Input: part model. Units: mm. Frame: model coordinates. A direction names the side the tool comes from. Give positions to 0.01 mm unless a question says otherwise; leave off trailing zeros. Loops run counter-clockwise (first coordinate to the right, second up) from the corner with the lowest first, then second, coordinate; pieces in that order, holes last. Notation, with made-up numbers: M 25,-13.75 L 56,-13.75 A10 ccw 56,-7.75 Z; hole C 21.25,53.5 d5. An arc over 180 degrees is marked long. One line per item, written item: value. Start each with the question number.
(1) Section C-C on y = -43. Output: boundary loops of the cut face in (x, z), plus the area to 3 significant figures.
(2) Ray query, line 1 along Z through (x, y) = (-49, -48.5); line 2 along X through (y, z) = (-38, -69.5); line 3 along Y through (x, z) = (35.5, 12.5). Return the intervals inside material, ascending. Write a range as from..to.
(3) Section D-D on y = -85.5. Output: boundary loops of the cut face in (x, z).
(4) Section B-B on x = 57.5. Output: boundary loops of the cut face in (y, z), plus the area to 3 significant figures.
(5) Section A-A on z = -60.5. Output: boundary loops of the cut face in (x, y), plus the area to 3 significant figures.
(6) Pin query (flat end, axial travel): P1, Ø3.5, axis at x = -70, z = -70.5, coming from the -Y side; P2, Ø5, axis at x = 2.66, y = -73.34, coming from the +Z side. Return the tip coordinate at first contact, or that it passes through.
(7) Pull-direction query (Y, two-part tool) for faces 1 (the flat face through (-69, -52.086, -56)), 2 (the flat face through (1, -70, -130)), 3 (the cylindrical face through (-3.626, -178.175, -120.14)), 4 (the cylindrical face through (48.677, -115.843, 9.86)); classes: released by +Y, released by -Y, zero draft, split by the parting line, or undercut.
(8) Access query for faces 5 (the flat face through (-1, -22.086, 13)), 6 (the flat face through (70, -195, 10)), 7 (the flat face through (1, -70, -110)), 8 (the flat face through (-63, -37, -54)), 9 (the flat face through (69, -52.086, -56)). Directions: +Z, -Z, +X, -X, +Y, -Y. A direction counts if a zero-diameter tool reaches every point of the face in a straight line with its end or side. Return the directions, or none.
```python
from build123d import *

# Parameters (mm, degrees)
EXTRUDE_1_OUTLINE_W     = 150
EXTRUDE_1_OUTLINE_H     = 400
EXTRUDE_1_OUTLINE_R     = 48.25
EXTRUDE_1_DEPTH         = 20
SKETCH_2_W              = 150
SKETCH_2_H              = 400
SKETCH_2_W_2            = 126
SKETCH_2_H_2            = 376
EXTRUDE_1_2_DEPTH       = 110
EXTRUDE_START           = 20
SKETCH_3_W              = 150
SKETCH_3_H              = 400
SKETCH_3_R              = 48.25
EXTRUDE_3_DEPTH         = 20
SKETCH_4_W              = 110
SKETCH_4_H              = 55
CUT_EXTRUDE_1_DEPTH     = 428.229446551
CHAMFER_2_SIZE          = 20
CHAMFER_3_SIZE          = 20
CUT_EXTRUDE_START       = 190
CUT_EXTRUDE_2_OUTLINE_W = 132
CUT_EXTRUDE_2_OUTLINE_H = 152
CUT_EXTRUDE_2_DEPTH     = 10
FILLET_1_R              = 20
FILLET_2_R              = 20
FILLET_3_R              = 20
FILLET_4_R              = 20
EXTRUDE_START_2         = -20
SKETCH_6_R              = 48.25
SKETCH_6_R_2            = 29.5
EXTRUDE_4_DEPTH         = 20
SKETCH_7_R              = 48.25
SKETCH_7_R_2            = 29.5
EXTRUDE_5_DEPTH         = 20
SKETCH_8_R              = 29.5
EXTRUDE_7_DEPTH         = 20
SKETCH_9_R              = 29.5
EXTRUDE_8_DEPTH         = 20
SKETCH_10_R             = 1.65
EXTRUDE_9_DEPTH         = 10
EXTRUDE_START_3         = 10
SKETCH_11_R             = 1.65
EXTRUDE_10_DEPTH        = 10
SKETCH_12_W             = 110
SKETCH_12_H             = 147.914448675
CUT_EXTRUDE_3_DEPTH     = 287.530975638
CHAMFER_4_SIZE          = 10
CHAMFER_5_SIZE          = 10
SKETCH_13_W             = 150
SKETCH_13_H             = 80
CUT_EXTRUDE_5_DEPTH     = 267.880122902
CUT_EXTRUDE_6_REACH     = 263.008
SKETCH_15_R             = 1.5
SKETCH_16_R             = 1.5
CUT_EXTRUDE_7_DEPTH     = 262.007662723


with BuildPart() as part:
    # Extrude 1: read off the stored shape, not the designer's step
    # Extrude 1 outline → Extrude 1 (new body)
    with BuildSketch(Plane.XY):
        Rectangle(EXTRUDE_1_OUTLINE_W, EXTRUDE_1_OUTLINE_H)
        with Locations((2.655190842, -130.335551325)):
            Circle(EXTRUDE_1_OUTLINE_R, mode=Mode.SUBTRACT)
        with Locations((0, 129.13990983)):
            Circle(EXTRUDE_1_OUTLINE_R, mode=Mode.SUBTRACT)
    extrude(amount=EXTRUDE_1_DEPTH)

    # 草图2 → Extrude 1 2 (add)
    with BuildSketch(Plane(origin=(0, 0, 0), x_dir=(-1, 0, 0), z_dir=(0, 0, -1))):
        Rectangle(SKETCH_2_W, SKETCH_2_H)
        Rectangle(SKETCH_2_W_2, SKETCH_2_H_2, mode=Mode.SUBTRACT)
    extrude(amount=EXTRUDE_1_2_DEPTH)

    # 草图3 → 凸台-拉伸3 (add)
    with BuildSketch(Plane(origin=(0, 0, -110), x_dir=(-1, 0, 0), z_dir=(0, 0, -1)).offset(EXTRUDE_START)):
        Rectangle(SKETCH_3_W, SKETCH_3_H)
        with Locations(Location((-2.655190842, -130.335551325, 0), (0, 0, 180))):
            Circle(SKETCH_3_R, mode=Mode.SUBTRACT)
        with Locations(Location((0, 129.13990983, 0), (0, 0, 180))):
            Circle(SKETCH_3_R, mode=Mode.SUBTRACT)
    extrude(amount=-EXTRUDE_3_DEPTH)

    # 草图4 → 切除-拉伸1 (cut, through all)
    with BuildSketch(Plane.XZ.offset(200)):
        with Locations((0, -27.5)):
            Rectangle(SKETCH_4_W, SKETCH_4_H)
        with Locations((0, -82.5)):
            Rectangle(SKETCH_4_W, SKETCH_4_H)
    extrude(amount=-CUT_EXTRUDE_1_DEPTH, mode=Mode.SUBTRACT)

    # 倒角2
    chamfer_2_edges = [part.edges().sort_by_distance(p)[0] for p in [
        (-75, 200, -55),
    ]]
    chamfer(chamfer_2_edges, length=CHAMFER_2_SIZE - 0.0001)  # a hair under: the kernel refuses the full size

    # 倒角3
    chamfer_3_edges = [part.edges().sort_by_distance(p)[0] for p in [
        (75, 200, -55),
    ]]
    chamfer(chamfer_3_edges, length=CHAMFER_3_SIZE - 0.0001)  # a hair under: the kernel refuses the full size

    # 切除-拉伸2: read off the stored shape, not the designer's step
    # 切除-拉伸2 outline → 切除-拉伸2 (cut)
    with BuildSketch(Plane(origin=(0, 0, 0), x_dir=(1, 0, 0), z_dir=(0, 1, 0)).offset(CUT_EXTRUDE_START)):
        with Locations((0, 55)):
            Rectangle(CUT_EXTRUDE_2_OUTLINE_W, CUT_EXTRUDE_2_OUTLINE_H)
    extrude(amount=CUT_EXTRUDE_2_DEPTH, mode=Mode.SUBTRACT)

    # 圆角1
    fillet_1_edges = [part.edges().sort_by_distance(p)[0] for p in [
        (-65.0001, 190, -55),
    ]]
    fillet(fillet_1_edges, radius=FILLET_1_R)

    # 圆角2
    fillet_2_edges = [part.edges().sort_by_distance(p)[0] for p in [
        (65.0001, 190, -55),
    ]]
    fillet(fillet_2_edges, radius=FILLET_2_R)

    # 圆角3
    # the kernel refuses this fillet: 20 mm, written as the material it takes off along each edge
    with BuildSketch(Plane(origin=(-75, 180.0001, 40.112615753), x_dir=(0.7071067811865488, 0.7071067811865464, 0), z_dir=(0, 0, -1))) as fillet_3_piece_1:
        with BuildLine():
            CenterArc((8.453428829, 19.830842418), FILLET_3_R, 225, 37.542814558)
            Line((-5.688706794, 5.688706794), (-5.971549507, 5.405864082))
            Line((-5.971549507, 5.405864082), (-0.282842712, -0.282842712))
            Line((-0.282842712, -0.282842712), (0, -0.4))
            ThreePointArc((0, -0.4), (2.928861477, -0.4), (5.805808837, -0.396616848))
            Line((5.805808837, -0.396616848), (5.857722955, 0))
        make_face()
    extrude(amount=190.225231505, mode=Mode.SUBTRACT)

    # 圆角4
    # the kernel refuses this fillet: 20 mm, written as the material it takes off along each edge
    with BuildSketch(Plane(origin=(75, 180.0001, -150.112615753), x_dir=(-0.7071067811865438, 0.7071067811865511, 0), z_dir=(0, 0, 1))) as fillet_4_piece_1:
        with BuildLine():
            CenterArc((8.453428829, 19.830842418), FILLET_4_R, 225, 37.542814558)
            Line((-5.688706794, 5.688706794), (-5.971549507, 5.405864082))
            Line((-5.971549507, 5.405864082), (-0.282842712, -0.282842712))
            Line((-0.282842712, -0.282842712), (0, -0.4))
            ThreePointArc((0, -0.4), (2.928861477, -0.4), (5.805808837, -0.396616848))
            Line((5.805808837, -0.396616848), (5.857722955, 0))
        make_face()
    extrude(amount=190.225231505, mode=Mode.SUBTRACT)

    # 草图6 → 凸台-拉伸4 (add)
    with BuildSketch(Plane.XY.offset(20).offset(EXTRUDE_START_2)):
        with Locations(Location((0, 129.13990983, 0), (0, 0, 180))):
            Circle(SKETCH_6_R)
        with Locations((0, 129.13990983)):
            Circle(SKETCH_6_R_2, mode=Mode.SUBTRACT)
    extrude(amount=EXTRUDE_4_DEPTH)

    # 草图7 → 凸台-拉伸5 (add)
    with BuildSketch(Plane(origin=(0, 0, -130), x_dir=(-1, 0, 0), z_dir=(0, 0, -1))):
        with Locations((0, 129.13990983)):
            Circle(SKETCH_7_R)
        with Locations(Location((0, 129.13990983, 0), (0, 0, 180))):
            Circle(SKETCH_7_R_2, mode=Mode.SUBTRACT)
    extrude(amount=-EXTRUDE_5_DEPTH)

    # 草图8 → 凸台-拉伸7 (add)
    with BuildSketch(Plane.XY.offset(20).offset(EXTRUDE_START_2)):
        with Locations(Location((0, 129.13990983, 0), (0, 0, 180))):
            Circle(SKETCH_8_R)
    extrude(amount=EXTRUDE_7_DEPTH)

    # 草图9 → 凸台-拉伸8 (add)
    with BuildSketch(Plane(origin=(0, 0, -130), x_dir=(-1, 0, 0), z_dir=(0, 0, -1))):
        with Locations((0, 129.13990983)):
            Circle(SKETCH_9_R)
    extrude(amount=-EXTRUDE_8_DEPTH)

    # 草图10 → 凸台-拉伸9 (add)
    with BuildSketch(Plane(origin=(0, 0, -130), x_dir=(-1, 0, 0), z_dir=(0, 0, -1))):
        with Locations((0, 146.38990983)):
            Circle(SKETCH_10_R)
        with Locations((14.938938215, 137.76490983)):
            Circle(SKETCH_10_R)
        with Locations((14.938938215, 120.51490983)):
            Circle(SKETCH_10_R)
        with Locations((0, 111.88990983)):
            Circle(SKETCH_10_R)
        with Locations((-14.938938215, 120.51490983)):
            Circle(SKETCH_10_R)
        with Locations((-14.938938215, 137.76490983)):
            Circle(SKETCH_10_R)
    extrude(amount=EXTRUDE_9_DEPTH)

    # 草图11 → 凸台-拉伸10 (add)
    with BuildSketch(Plane.XY.offset(20).offset(EXTRUDE_START_3)):
        with Locations(Location((-14.938938215, 137.76490983, 0), (0, 0, 180))):
            Circle(SKETCH_11_R)
        with Locations(Location((-14.938938215, 120.51490983, 0), (0, 0, 180))):
            Circle(SKETCH_11_R)
        with Locations(Location((0, 111.88990983, 0), (0, 0, 180))):
            Circle(SKETCH_11_R)
        with Locations(Location((14.938938215, 120.51490983, 0), (0, 0, 180))):
            Circle(SKETCH_11_R)
        with Locations(Location((0, 146.38990983, 0), (0, 0, 180))):
            Circle(SKETCH_11_R)
        with Locations(Location((14.938938215, 137.76490983, 0), (0, 0, 180))):
            Circle(SKETCH_11_R)
    extrude(amount=-EXTRUDE_10_DEPTH)

    # 草图12 → 切除-拉伸3 (cut, through all)
    with BuildSketch(Plane.ZY.offset(75)):
        with Locations((-55, -126.042775663)):
            Rectangle(SKETCH_12_W, SKETCH_12_H)
    extrude(amount=-CUT_EXTRUDE_3_DEPTH, mode=Mode.SUBTRACT)

    # 倒角4
    chamfer_4_edges = [part.edges().sort_by_distance(p)[0] for p in [
        (-75, -200, -120),
    ]]
    chamfer(chamfer_4_edges, length=CHAMFER_4_SIZE)

    # 倒角5
    chamfer_5_edges = [part.edges().sort_by_distance(p)[0] for p in [
        (75, -200, -120),
        (-75, -200, 10),
        (75, -200, 10),
    ]]
    chamfer(chamfer_5_edges, length=CHAMFER_5_SIZE)

    # 草图13 → 切除-拉伸5 (cut, through all)
    with BuildSketch(Plane.XY.offset(20)):
        with Locations((0, 17.914448675)):
            Rectangle(SKETCH_13_W, SKETCH_13_H)
    extrude(amount=-CUT_EXTRUDE_5_DEPTH, mode=Mode.SUBTRACT)


with BuildPart() as body_2:
    # of the pieces the cut leaves, the one that is kept (cut_extrude_5_keep)
    add(part.part.solids().sort_by_distance((65, -200, -110))[0])

    # 草图15 → 切除-拉伸6 (cut, up to next)
    with BuildSketch(Plane.XY.offset(20), mode=Mode.PRIVATE) as cut_extrude_6_sk1:
        with Locations((2.655190842, -73.335551325)):
            Circle(SKETCH_15_R)
    cut_extrude_6_tool1 = extrude(cut_extrude_6_sk1.sketch, amount=-CUT_EXTRUDE_6_REACH, mode=Mode.PRIVATE) & body_2.part
    # 草图15 → 切除-拉伸6 (cut, up to next)
    with BuildSketch(Plane.XY.offset(20), mode=Mode.PRIVATE) as cut_extrude_6_sk2:
        with Locations((52.018638858, -101.835551325)):
            Circle(SKETCH_15_R)
    cut_extrude_6_tool2 = extrude(cut_extrude_6_sk2.sketch, amount=-CUT_EXTRUDE_6_REACH, mode=Mode.PRIVATE) & body_2.part
    # 草图15 → 切除-拉伸6 (cut, up to next)
    with BuildSketch(Plane.XY.offset(20), mode=Mode.PRIVATE) as cut_extrude_6_sk3:
        with Locations((52.018638858, -158.835551325)):
            Circle(SKETCH_15_R)
    cut_extrude_6_tool3 = extrude(cut_extrude_6_sk3.sketch, amount=-CUT_EXTRUDE_6_REACH, mode=Mode.PRIVATE) & body_2.part
    # 草图15 → 切除-拉伸6 (cut, up to next)
    with BuildSketch(Plane.XY.offset(20), mode=Mode.PRIVATE) as cut_extrude_6_sk4:
        with Locations((2.655190842, -187.335551325)):
            Circle(SKETCH_15_R)
    cut_extrude_6_tool4 = extrude(cut_extrude_6_sk4.sketch, amount=-CUT_EXTRUDE_6_REACH, mode=Mode.PRIVATE) & body_2.part
    # 草图15 → 切除-拉伸6 (cut, up to next)
    with BuildSketch(Plane.XY.offset(20), mode=Mode.PRIVATE) as cut_extrude_6_sk5:
        with Locations((-46.708257174, -158.835551325)):
            Circle(SKETCH_15_R)
    cut_extrude_6_tool5 = extrude(cut_extrude_6_sk5.sketch, amount=-CUT_EXTRUDE_6_REACH, mode=Mode.PRIVATE) & body_2.part
    # 草图15 → 切除-拉伸6 (cut, up to next)
    with BuildSketch(Plane.XY.offset(20), mode=Mode.PRIVATE) as cut_extrude_6_sk6:
        with Locations((-46.708257174, -101.835551325)):
            Circle(SKETCH_15_R)
    cut_extrude_6_tool6 = extrude(cut_extrude_6_sk6.sketch, amount=-CUT_EXTRUDE_6_REACH, mode=Mode.PRIVATE) & body_2.part
    add(cut_extrude_6_tool1.solids().sort_by_distance((2.655191, -73.335551, 20))[0], mode=Mode.SUBTRACT)
    add(cut_extrude_6_tool2.solids().sort_by_distance((52.018639, -101.835551, 20))[0], mode=Mode.SUBTRACT)
    add(cut_extrude_6_tool3.solids().sort_by_distance((52.018639, -158.835551, 20))[0], mode=Mode.SUBTRACT)
    add(cut_extrude_6_tool4.solids().sort_by_distance((2.655191, -187.335551, 20))[0], mode=Mode.SUBTRACT)
    add(cut_extrude_6_tool5.solids().sort_by_distance((-46.708257, -158.835551, 20))[0], mode=Mode.SUBTRACT)
    add(cut_extrude_6_tool6.solids().sort_by_distance((-46.708257, -101.835551, 20))[0], mode=Mode.SUBTRACT)

    # 草图16 → 切除-拉伸7 (cut, through all)
    with BuildSketch(Plane(origin=(0, 0, -130), x_dir=(-1, 0, 0), z_dir=(0, 0, -1))):
        with Locations(Location((-52.018638858, -101.835551325, 0), (0, 0, 180))):
            Circle(SKETCH_16_R)
        with Locations(Location((-2.655190842, -73.335551325, 0), (0, 0, 180))):
            Circle(SKETCH_16_R)
        with Locations(Location((46.708257174, -158.835551325, 0), (0, 0, 180))):
            Circle(SKETCH_16_R)
        with Locations(Location((-52.018638858, -158.835551325, 0), (0, 0, 180))):
            Circle(SKETCH_16_R)
        with Locations(Location((-2.655190842, -187.335551325, 0), (0, 0, 180))):
            Circle(SKETCH_16_R)
        with Locations(Location((46.708257174, -101.835551325, 0), (0, 0, 180))):
            Circle(SKETCH_16_R)
    extrude(amount=-CUT_EXTRUDE_7_DEPTH, mode=Mode.SUBTRACT)


solid = body_2.part
```
Output values:
1. outline: M -75,-130 L 75,-130 L 75,20 L -75,20 Z; hole M -63,-110 L 63,-110 L 63,0 L -63,0 Z
1. area: 8,640 mm²
2. line 1: z = -130..-110, 0..20
2. line 2: x = -75..-63, 63..75
2. line 3: y = -200..-165.68, -94.99..-22.09
3. outline: M -75,-130 L -15.17,-130 L -15.17,-110 L -75,-110 Z; M -75,0 L -15.17,0 L -15.17,20 L -75,20 Z; M 20.48,-130 L 75,-130 L 75,-110 L 20.48,-110 Z; M 20.48,0 L 75,0 L 75,20 L 20.48,20 Z
4. outline: M -200,-130 L -22.09,-130 L -22.09,-110 L -200,-110 Z; M -200,0 L -22.09,0 L -22.09,20 L -200,20 Z
4. area: 7,120 mm²
5. outline: M -75,-52.09 L -63,-52.09 L -63,-22.09 L -75,-22.09 Z; M 63,-52.09 L 75,-52.09 L 75,-22.09 L 63,-22.09 Z
5. area: 720 mm²
6. P1: stops at y = -52.09
6. P2: stops at z = 20
7. face 1: released by -Y
7. face 2: zero draft
7. face 3: undercut
7. face 4: undercut
8. face 5: +Z, -Z, +X, -X, +Y
8. face 6: +Z, -Z, +X, -Y
8. face 7: -Y
8. face 8: +Y, -Y
8. face 9: +X, -X, -Y
